Study the drawing (mm; zero at the part's minimum x, y, z) and answer. A direction names the side the tool comes from. Give positions to 0.01 mm unless a question says otherwise; leave off trailing zeros. Write each loop counter-clockwise with the first axis right and the second up, starting at its lowest first coordinate (ties: lowest second). Pieces come first, ordered by that corner, then holes. Notation, with made-up numbers: (55.25, -37) -> (95.25, -37) arc R29 ccw to (95.25, -17) -> close; hole circle Ø8 at (52.25, 73.25). An arc over 180 degrees is marked (long way). One line per question, with ' | ' between items.
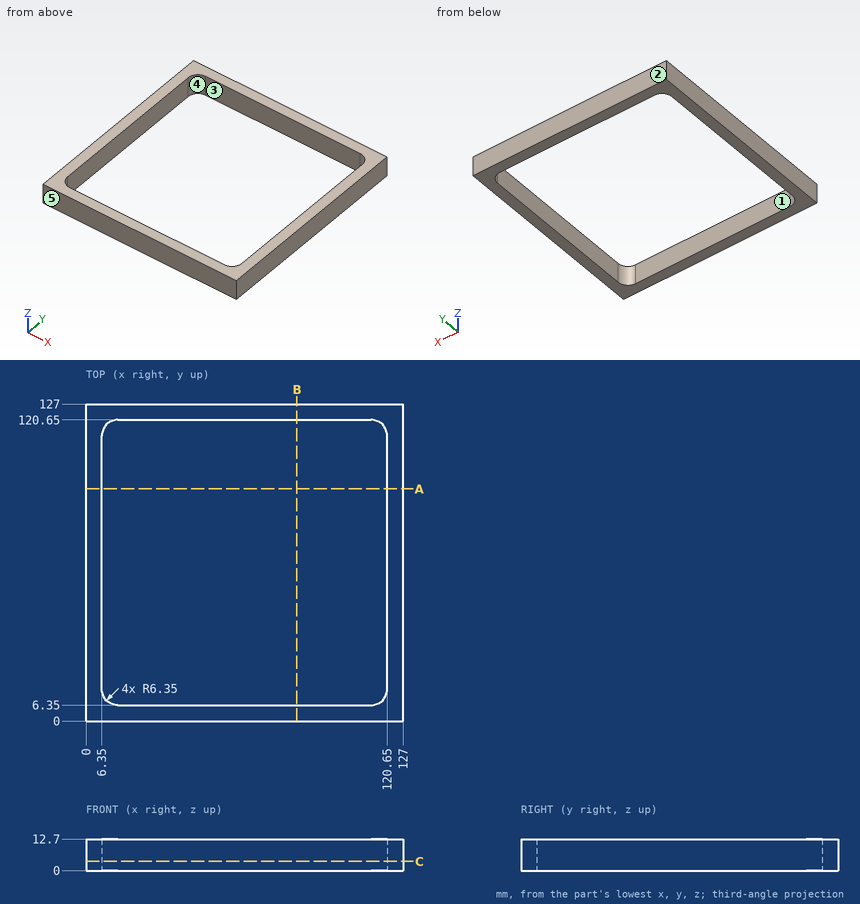
Item 1: Determine the mould class of the marked faces 1, 2 and 3 for opening direction X: pulls with the +X half, pulls with the -X half, needs draft (parallel to the pull), parting line crosses it, or undercut.
Answers below:
face 1: undercut | face 2: needs draft | face 3: undercut
Item 2: Find section A-A (y = 93). Write down the section's boundary in (x, z).
Answers below:
outline: (0, 0) -> (6.35, 0) -> (6.35, 12.7) -> (0, 12.7) -> close; (120.65, 0) -> (127, 0) -> (127, 12.7) -> (120.65, 12.7) -> close
Item 3: Consider line 1 (X direction, y = 64, z = 11); line 2 (X direction, y = 119, z = 8). Determine where each line is inside the solid, lowest interval first. Write a range as [from, to].
Answers below:
line 1: [0, 6.35], [120.65, 127] | line 2: [0, 8.43], [118.57, 127]
Item 4: A flat-ended cylindrical pin translates along its axis: pin 1 (3 mm diameter, centred on y = 64, z = 3.5, fed in from -X). Find the tip coordinate at first contact, or state that the pin passes through.
Answers below:
pin 1: x = 0
Item 5: A tool of negligible diameter and unlimited length cuts with its end or side. For the marked faces 4 and 5, from which of +Z, -Z, +X, -X, +Y, -Y can it reach the whole face along a straight path? Write none if from no direction.
Answers below:
face 4: +Z, -Z | face 5: +Z, -Z, +X, -X, -Y
Item 6: Find section C-C (z = 3.75). Write down the section's boundary in (x, y), then the cut area to 3 significant figures.
Answers below:
outline: (0, 0) -> (127, 0) -> (127, 127) -> (0, 127) -> close; hole (6.35, 12.7) arc R6.35 ccw to (12.7, 6.35) -> (114.3, 6.35) arc R6.35 ccw to (120.65, 12.7) -> (120.65, 114.3) arc R6.35 ccw to (114.3, 120.65) -> (12.7, 120.65) arc R6.35 ccw to (6.35, 114.3) -> close | area: 3,100 mm²
